from build123d import *

# Parameters (mm, degrees)
SKETCH1_W           = 134
SKETCH1_H           = 40
SKETCH1_R           = 2.85
BOSS_EXTRUDE1_DEPTH = 15
SKETCH2_R           = 5
CUT_EXTRUDE1_DEPTH  = 2
FILLET1_R           = 3


with BuildPart() as part:
    # Sketch1 → Boss-Extrude1 (new body)
    with BuildSketch(Plane.XY):
        Rectangle(SKETCH1_W, SKETCH1_H)
        with Locations((-51, 10)):
            Circle(SKETCH1_R, mode=Mode.SUBTRACT)
        with Locations((-17, 10)):
            Circle(SKETCH1_R, mode=Mode.SUBTRACT)
        with Locations((17, 10)):
            Circle(SKETCH1_R, mode=Mode.SUBTRACT)
        with Locations((51, 10)):
            Circle(SKETCH1_R, mode=Mode.SUBTRACT)
        with Locations((-17, -10)):
            Circle(SKETCH1_R, mode=Mode.SUBTRACT)
        with Locations((17, -10)):
            Circle(SKETCH1_R, mode=Mode.SUBTRACT)
        with Locations((51, -10)):
            Circle(SKETCH1_R, mode=Mode.SUBTRACT)
        with Locations((-51, -10)):
            Circle(SKETCH1_R, mode=Mode.SUBTRACT)
    extrude(amount=BOSS_EXTRUDE1_DEPTH)

    # Sketch2 → Cut-Extrude1 (cut)
    with BuildSketch(Plane.XY.offset(15)):
        with Locations((-51, 10)):
            Circle(SKETCH2_R)
        with Locations((-17, 10)):
            Circle(SKETCH2_R)
        with Locations((17, 10)):
            Circle(SKETCH2_R)
        with Locations((51, 10)):
            Circle(SKETCH2_R)
        with Locations((-17, -10)):
            Circle(SKETCH2_R)
        with Locations((17, -10)):
            Circle(SKETCH2_R)
        with Locations((51, -10)):
            Circle(SKETCH2_R)
        with Locations((-51, -10)):
            Circle(SKETCH2_R)
    extrude(amount=-CUT_EXTRUDE1_DEPTH, mode=Mode.SUBTRACT)

    # Fillet1
    fillet1_edges = [part.edges().sort_by_distance(p)[0] for p in [
        (-67, 0, 15),
        (0, -20, 15),
        (67, 0, 15),
        (67, -20, 7.5),
        (-67, -20, 7.5),
        (-67, 20, 7.5),
        (67, 20, 7.5),
        (0, 20, 15),
    ]]
    fillet(fillet1_edges, radius=FILLET1_R)


solid = part.part
Input: part model. Units: mm. Frame: model coordinates. A direction names the side the tool comes from. Give positions to 0.01 mm unless a question says otherwise; leave off trailing zeros. Order: outer loops, then holes, each group sorted by start corner. A loop starts at its lowest first (then second) coordinate and runs counter-clockwise, first axis right, second up. Notation, with made-up numbers: (85, 41) - (105, 41) arc R32 ccw to (105, 67) - close; hole circle Ø2 at (69, 18.5). An arc over 180 degrees is marked (long way). Answer as a JSON object with one key per item and string values. Group by question number.
Q1. Mould query, pull axis Y, two halves, no side actions, for faces 3 (the face through (21.77, 11.5, 14.01)), 4 (the face through (0.9, 19.14, 14.1)), 5 (the face through (-1, -20, 6)). Classes: pulls with the +Y half, pulls with the -Y half, needs draft (parallel to the pull), parting line crosses it, or undercut.
Q2. Cut plane B-B, the plane z = 5. Count the separate pieces of the cut face and the enclosed holes in it, then the cut area to 3 significant figures.
Q3. First-contact query: pin 1 Ø3 at (x, y) = (51, 12) entering from +Z. Flat tip, straight axial feed; report the tip coordinate or a pass-through.
Q4. Set-up query: faces 1 (the face through (-67, 0, 6)), 2 (the face through (-21, -7, 14)). Return all of +Z, -Z, +X, -X, +Y, -Y with unobstructed straight access to the full face (end or side cutting, diameter ignored); none if empty.
Q5. Line query: probe 1 along X at (y, z) = (-12.5, 12.25); probe 2 along Y at (x, z) = (17, 14.45); probe 3 along Y at (x, z) = (19, 10). Output: solid intervals per line, ascending.
Q6. Cut plane A-A, the plane x = -51. Output: boundary loops of the cut face in (y, z), then the cut area to 3 significant figures.
Results:
{
 "1": {"face 3": "undercut", "face 4": "pulls with the +Y half", "face 5": "pulls with the -Y half"},
 "2": {"separate pieces": "1", "enclosed holes": "8", "area": "5,150 mm^2"},
 "3": {"pin 1": "z = 13"},
 "4": {"face 1": "+Z, -Z, -X, +Y, -Y", "face 2": "+Z"},
 "5": {"probe 1": "-66.99 to -52.37, -49.63 to -18.37, -15.63 to 15.63, 18.37 to 49.63, 52.37 to 66.99", "probe 2": "-18.73 to -15, -5 to 5, 15 to 18.73", "probe 3": "-20 to -12.03, -7.97 to 7.97, 12.03 to 20"},
 "6": {"outline": "(-20, 0) - (-12.85, 0) - (-12.85, 13) - (-15, 13) - (-15, 15) - (-17, 15) arc R3 ccw to (-20, 12) - close; (-7.15, 0) - (7.15, 0) - (7.15, 13) - (5, 13) - (5, 15) - (-5, 15) - (-5, 13) - (-7.15, 13) - close; (12.85, 0) - (20, 0) - (20, 12) arc R3 ccw to (17, 15) - (15, 15) - (15, 13) - (12.85, 13) - close", "area": "408 mm^2"}
}
